Design review of the part built by this model. Coordinates are the model's own, in mm. A direction names the side the tool comes from. Round coordinates to 2 decimals unless told otherwise and drop trailing zeros. Write each loop counter-clockwise with the first axis right and the second up, starting at its lowest first coordinate (ties: lowest second). Pieces come first, ordered by that corner, then holes.
from build123d import *

# Parameters (mm, degrees)
BOSS_EXTRUDE1_DEPTH                             = 15.4
CUT_EXTRUDE2_REACH                              = 25.918
SKETCH3_W                                       = 7
SKETCH3_H                                       = 11.5
BOSS_EXTRUDE3_REACH                             = 25.918
SKETCH4_W                                       = 0.8
SKETCH4_H                                       = 6.2
SKETCH4_W_2                                     = 2.8
SKETCH4_H_2                                     = 17.7
SKETCH10_W                                      = 4
SKETCH10_H                                      = 0.7
CUT_EXTRUDE4_DEPTH                              = 16.3
BOSS_EXTRUDE4_DEPTH                             = 0.8
CSK_FOR_M2_FLAT_HEAD_MACHINE_SCREW3_D           = 2.4
CSK_FOR_M2_FLAT_HEAD_MACHINE_SCREW3_CSINK_D     = 4.4
CSK_FOR_M2_FLAT_HEAD_MACHINE_SCREW3_CSINK_ANGLE = 90
MOVE_FACE1_BY                                   = 0.6
FILLET3_R                                       = 0.8
CHAMFER1_SIZE                                   = 2.5
CHAMFER1_SIZE2                                  = 4
SKETCH12_W                                      = 2.0475
SKETCH12_H                                      = 3.18
BOSS_EXTRUDE5_DEPTH                             = 17.7
FILLET5_R                                       = 0.5
SKETCH11_R                                      = 1.75
CUT_EXTRUDE5_DEPTH                              = 25.492262043
CUT_EXTRUDE5_DIRECTION_2_REACH                  = 26.492


with BuildPart() as part:
    # Sketch2 → Boss-Extrude1 (new body)
    with BuildSketch(Plane(origin=(0, 0, 0), x_dir=(0, 0, -1), z_dir=(1, 0, 0))):
        Polygon((0, 0), (-4.65, 0), (-4.65, 17.7), (-3.85, 17.7), (-3.85, 0.8), (-0.7, 0.8), (-0.7, 17.7), (0, 17.7), align=None)
    extrude(amount=BOSS_EXTRUDE1_DEPTH)

    # Sketch3 → Cut-Extrude2 (cut, up to next)
    with BuildSketch(Plane.XY.offset(4.65), mode=Mode.PRIVATE) as cut_extrude2_sk1:
        with Locations((3.5, 11.95)):
            Rectangle(SKETCH3_W, SKETCH3_H)
    cut_extrude2_tool1 = extrude(cut_extrude2_sk1.sketch, amount=-CUT_EXTRUDE2_REACH, mode=Mode.PRIVATE) & part.part
    add(cut_extrude2_tool1.solids().sort_by_distance((3.5, 11.95, 4.65))[0], mode=Mode.SUBTRACT)

    # Sketch4 → Boss-Extrude3 (add, up to next)
    with BuildSketch(Plane.XY.offset(4.65), mode=Mode.PRIVATE) as boss_extrude3_sk1:
        with Locations((0.4, 3.1)):
            Rectangle(SKETCH4_W, SKETCH4_H)
    boss_extrude3_tool1 = extrude(boss_extrude3_sk1.sketch, amount=-BOSS_EXTRUDE3_REACH, mode=Mode.PRIVATE) - part.part
    # Sketch4 → Boss-Extrude3 (add, up to next)
    with BuildSketch(Plane.XY.offset(4.65), mode=Mode.PRIVATE) as boss_extrude3_sk2:
        with Locations((14, 8.85)):
            Rectangle(SKETCH4_W_2, SKETCH4_H_2)
    boss_extrude3_tool2 = extrude(boss_extrude3_sk2.sketch, amount=-BOSS_EXTRUDE3_REACH, mode=Mode.PRIVATE) - part.part
    add(boss_extrude3_tool1.solids().sort_by_distance((0.4, 3.1, 4.65))[0])
    add(boss_extrude3_tool2.solids().sort_by_distance((14, 8.85, 4.65))[0])

    # Sketch10 → Cut-Extrude4 (cut)
    with BuildSketch(Plane(origin=(0, 17.7, 0), x_dir=(1, 0, 0), z_dir=(0, 1, 0))):
        with Locations((10.2, -0.35)):
            Rectangle(SKETCH10_W, SKETCH10_H)
    extrude(amount=-CUT_EXTRUDE4_DEPTH, mode=Mode.SUBTRACT)

    # Sketch6 → Boss-Extrude4 (add)
    with BuildSketch(Plane(origin=(0, 0, 3.85), x_dir=(-1, 0, 0), z_dir=(0, 0, -1))):
        with BuildLine():
            Line((-0.8, 0.8), (-5.05, 0.8))
            Line((-5.05, 0.8), (-5.05, 2.95))
            ThreePointArc((-5.05, 2.95), (-4.508147545, 4.258147545), (-3.2, 4.8))
            Line((-3.2, 4.8), (-0.8, 4.8))
            Line((-0.8, 4.8), (-0.8, 0.8))
        make_face()
    extrude(amount=BOSS_EXTRUDE4_DEPTH)

    # CSK for M2 Flat Head Machine Screw3 (through all)
    with Locations(Plane(origin=(10.2, 14.95, 4.65), x_dir=(0, 1, 0), z_dir=(0, 0, 1))):
        with Locations((0, 0), (-12, 7)):
            CounterSinkHole(CSK_FOR_M2_FLAT_HEAD_MACHINE_SCREW3_D / 2, CSK_FOR_M2_FLAT_HEAD_MACHINE_SCREW3_CSINK_D / 2, counter_sink_angle=CSK_FOR_M2_FLAT_HEAD_MACHINE_SCREW3_CSINK_ANGLE)

    # Move Face1: a face moved inward by 0.6
    extrude(part.faces().sort_by_distance((4.1, 17.7, 0.35))[0], amount=MOVE_FACE1_BY, dir=(0, -1, 0), mode=Mode.SUBTRACT)

    # Fillet3
    fillet3_edges = [part.edges().sort_by_distance(p)[0] for p in [
        (0.8, 5.5, 3.85),
        (12.6, 9.25, 3.85),
        (0.4, 6.2, 0.7),
        (7, 6.2, 4.25),
        (7, 17.7, 4.25),
        (0, 17.1, 0.35),
    ]]
    fillet(fillet3_edges, radius=FILLET3_R)

    # Chamfer1
    chamfer1_edges = [part.edges().sort_by_distance(p)[0] for p in [
        (15.4, 8.85, 4.65),
    ]]
    chamfer1_side = [part.faces().sort_by_distance(p)[0] for p in [
        (9.979105197, 7.278141181, 4.65),
    ]]
    chamfer(chamfer1_edges, length=CHAMFER1_SIZE, length2=CHAMFER1_SIZE2, reference=chamfer1_side[0])

    # Sketch12 → Boss-Extrude5 (add)
    with BuildSketch(Plane(origin=(0, 17.7, 0), x_dir=(1, 0, 0), z_dir=(0, 1, 0))):
        with Locations((14.37625, 1.59)):
            Rectangle(SKETCH12_W, SKETCH12_H)
    extrude(amount=-BOSS_EXTRUDE5_DEPTH)

    # Fillet5
    fillet5_edges = [part.edges().sort_by_distance(p)[0] for p in [
        (12.9, 8.85, 4.65),
    ]]
    fillet(fillet5_edges, radius=FILLET5_R)

    # Sketch11 → Cut-Extrude5 (cut)
    with BuildSketch(Plane(origin=(0, 0, 3.85), x_dir=(-1, 0, 0), z_dir=(0, 0, -1))):
        with Locations(Location((-10.2, 14.95, 0), (0, 0, 270))):
            Circle(SKETCH11_R)
    extrude(amount=-CUT_EXTRUDE5_DEPTH, mode=Mode.SUBTRACT)

    # Sketch11 → Cut-Extrude5 direction 2 (cut, up to next)
    with BuildSketch(Plane(origin=(0, 0, 3.85), x_dir=(-1, 0, 0), z_dir=(0, 0, -1)), mode=Mode.PRIVATE) as cut_extrude5_direction_2_sk1:
        with Locations(Location((-10.2, 14.95, 0), (0, 0, 270))):
            Circle(SKETCH11_R)
    cut_extrude5_direction_2_tool1 = extrude(cut_extrude5_direction_2_sk1.sketch, amount=CUT_EXTRUDE5_DIRECTION_2_REACH, mode=Mode.PRIVATE) & part.part
    add(cut_extrude5_direction_2_tool1.solids().sort_by_distance((10.2, 14.95, 3.85))[0], mode=Mode.SUBTRACT)


solid = part.part
1) For faces 1 (the face through (8.465, 15.178, 4.015)), 2 (the face through (7.23, 17.46, 4.24)), 3 (the face through (5.05, 1.9, 3.5)), list the 3-axis set-ups (+Z, -Z, +X, -X, +Y, -Y) from which the entire face can be reached by the end or side of a thin tool; tool diameter is ignored.
2) Add section A-A on y = 14.95. Count the separate pieces of the cut face and the enclosed holes in it, and give its area (3 significant figures).
3) For P1, Ø1.9, axis at x = 3.2, y = 2.95, coming from the +Z side; P2, Ø0.9, axis at x = 1.5, z = 3.5, coming from the +Y side; P3, Ø0.7, axis at y = 3.5, z = 2.5, coming from the +X side; P4, Ø0.9, axis at y = 2.5, z = 3.5, coming from the +X side, all flat-tipped, find the tip position at first contact; note any pin that passes through.
4) Add section C-C on x = 10.2. State the section outline as (y, z) points, and give its area (3 significant figures).
5) Add section D-D on z = 2.75. State the section outline as (x, y) points.
6) For line 1 along X through (y, z) = (2.95, 0.3); line 2 along Y through (x, z) = (10.2, 4.05); line 3 along Z through (x, y) = (7.5, 6), list the stretches that pass through material, from the lowest coordinate up.
7) The part is to be moulded in two halves that separate along Z. For faces 4 (the face through (14, 9, -3.18)), 5 (the face through (4.265, 2.396, 0.345)), 6 (the face through (5, 9, 0.7)), 7 (the face through (2, 2, 3.05)), say which applies: pulls with the +Z half, pulls with the -Z half, needs draft (parallel to the pull), parting line crosses it, or undercut.
Computed:
1. face 1: +Z, -Z
1. face 2: +Z, -X, +Y
1. face 3: +Y
2. separate pieces: 3
2. enclosed holes: 0
2. area: 22.2 mm2
3. P1: passes through
3. P2: stops at y = 6.2
3. P3: stops at x = 14.46
3. P4: stops at x = 13.9
4. outline: (0, 0) - (1.4, 0) - (1.4, 0.7) - (0.8, 0.7) - (0.8, 3.85) - (13.2, 3.85) - (13.2, 4.2) - (12.75, 4.65) - (0, 4.65) - close; (16.7, 3.85) - (17.7, 3.85) - (17.7, 4.65) - (17.15, 4.65) - (16.7, 4.2) - close
4. area: 14.7 mm2
5. outline: (0, 0) - (14.09, 0) - (14.09, 17.7) - (12.6, 17.7) - (12.6, 0.8) - (0.8, 0.8) - (0.8, 6.2) - (0, 6.2) - close
6. line 1: x = 0 to 2, 4.4 to 8.2, 12.2 to 15.4
6. line 2: y = 0 to 13.2, 16.7 to 17.7
6. line 3: z = 0 to 0.7, 3.85 to 4.65
7. face 4: pulls with the -Z half
7. face 5: needs draft
7. face 6: undercut
7. face 7: undercut
